```python
from build123d import *

# Parameters (mm, degrees)
SKETCH_2_OUTSIDE_W        = 73.432
SKETCH_2_OUTSIDE_H        = 73.432
SKETCH_2_OUTSIDE_W_2      = 54
SKETCH_2_OUTSIDE_H_2      = 38
CUT_EXTRUDE_1_DEPTH       = 8
HOLE_WIZARD_1_D           = 5.5
HOLE_WIZARD_1_DEPTH       = 8
HOLE_WIZARD_1_CBORE_D     = 9.5
HOLE_WIZARD_1_CBORE_DEPTH = 5.4


with BuildPart() as part:
    # 草图1 → 旋转1 (revolve)
    with BuildSketch(Plane(origin=(0, 0, 0), x_dir=(0, 0, 1), z_dir=(0, -1, 0))):
        Polygon((0, 10), (42, 10), (42, 27), (34, 27), (34, 16), (0, 16), align=None)
    revolve(axis=Axis((0, 0, 0), (0, 0, 1)))

    # 草图2 outside → 切除-拉伸1 (cut)
    with BuildSketch(Plane.XY.offset(42)):
        Rectangle(SKETCH_2_OUTSIDE_W, SKETCH_2_OUTSIDE_H)
        Rectangle(SKETCH_2_OUTSIDE_W_2, SKETCH_2_OUTSIDE_H_2, mode=Mode.SUBTRACT)
    extrude(amount=-CUT_EXTRUDE_1_DEPTH, mode=Mode.SUBTRACT)

    # 孔1
    with Locations(Plane.XY.offset(42)):
        with Locations((-18, -12), (-18, 12), (18, 12), (18, -12), (0, 0)):
            CounterBoreHole(HOLE_WIZARD_1_D / 2, HOLE_WIZARD_1_CBORE_D / 2, HOLE_WIZARD_1_CBORE_DEPTH, depth=HOLE_WIZARD_1_DEPTH)


solid = part.part
```
Geometry check sheet. Reference: the model listing, model coordinates, mm. A direction names the side the tool comes from. Round coordinates to 2 decimals unless told otherwise and drop trailing zeros. Order: outer loops, then holes, each group sorted by start corner. A loop starts at its lowest first (then second) coordinate and runs counter-clockwise, first axis right, second up. Notation, with made-up numbers: (-34, 64.25) - (7, 64.25) arc R21 ccw to (7, 69.25) - close; hole circle Ø9 at (18.5, 85). An arc over 180 degrees is marked (long way). Use a Markdown table: item, result. Add a question column.
1) Section check D-D (x = 18). Record the cut outline in (y, z).
2) Gauge pin test, flat ends, axial feed: P1, Ø3, axis at x = -18, y = 11.5, coming from the +Z side; P2, Ø1.5, axis at y = 4.5, z = 19.5, coming from the -X side; P3, Ø11, axis at x = -18, y = -12, coming from the -Z side; P4, Ø7, axis at x = -18, y = -12, coming from the +Z side. Record the tip position at first contact, or that the pin passes through.
3) Thickness scan on line 1 along Y through (x, z) = (-18, 39.5); line 2 along Y through (x, z) = (0, 9); line 3 along X through (y, z) = (9, 26.5). Record the ranges inside material, lowest first.
4) Section check B-B (y = 0). Record the cut outline in (x, z), then the cut area to 3 significant figures.
5) Mould release check, pull along X, two halves, no side actions. Record for faces 1 (the flat face through (-12, -13, 34)), 2 (the cylindrical face through (-13.47, -10.57, 39.34)), 3 (the cylindrical face through (3.47, 15.62, 16.76)), 4 (the cylindrical face through (-27, 0, 38)): released by +X, released by -X, zero draft, split by the parting line, or undercut.
6) Section check C-C (z = 35.5). Record the cut outline in (x, y), then the cut area to 3 significant figures.
7) Set-up check for faces 5 (the flat face through (0, -19, 38)), 6 (the flat face through (21, 12, 36.6)): record each of +Z, -Z, +X, -X, +Y, -Y from which the full face is reachable in a straight line by a thin tool's end or side.
8) Section check A-A (x = 0). Record the cut outline in (y, z), then the cut area to 3 significant figures.
Established:
| question | item | result |
|---|---|---|
| 1 | outline | (-19, 34) - (-14.75, 34) - (-14.75, 36.6) - (-16.75, 36.6) - (-16.75, 42) - (-19, 42) - close; (-9.25, 34) - (9.25, 34) - (9.25, 36.6) - (7.25, 36.6) - (7.25, 42) - (-7.25, 42) - (-7.25, 36.6) - (-9.25, 36.6) - close; (14.75, 34) - (19, 34) - (19, 42) - (16.75, 42) - (16.75, 36.6) - (14.75, 36.6) - close |
| 2 | P1 | through |
| 2 | P2 | x = -15.55 |
| 2 | P3 | z = 34 |
| 2 | P4 | z = 36.6 |
| 3 | line 1 | -19 to -16.75, -7.25 to 7.25, 16.75 to 19 |
| 3 | line 2 | -16 to -10, 10 to 16 |
| 3 | line 3 | -13.23 to -4.36, 4.36 to 13.23 |
| 4 | outline | (-27, 34) - (-16, 34) - (-16, 0) - (-10, 0) - (-10, 42) - (-27, 42) - close; (10, 0) - (16, 0) - (16, 34) - (27, 34) - (27, 42) - (10, 42) - close |
| 4 | area | 680 mm2 |
| 5 | face 1 | zero draft |
| 5 | face 2 | undercut |
| 5 | face 3 | split by the parting line |
| 5 | face 4 | released by -X |
| 6 | outline | (-19.18, -19) - (19.18, -19) arc R27 ccw to (19.18, 19) - (-19.18, 19) arc R27 ccw to start; hole circle Ø5.5 at (-18, -12); hole circle Ø5.5 at (-18, 12); hole circle Ø20 at (0, 0); hole circle Ø5.5 at (18, -12); hole circle Ø5.5 at (18, 12) |
| 6 | area | 1,460 mm2 |
| 7 | face 5 | +Z, -Z, +X, -X, -Y |
| 7 | face 6 | +Z |
| 8 | outline | (-19, 34) - (-16, 34) - (-16, 0) - (-10, 0) - (-10, 42) - (-19, 42) - close; (10, 0) - (16, 0) - (16, 34) - (19, 34) - (19, 42) - (10, 42) - close |
| 8 | area | 552 mm2 |
